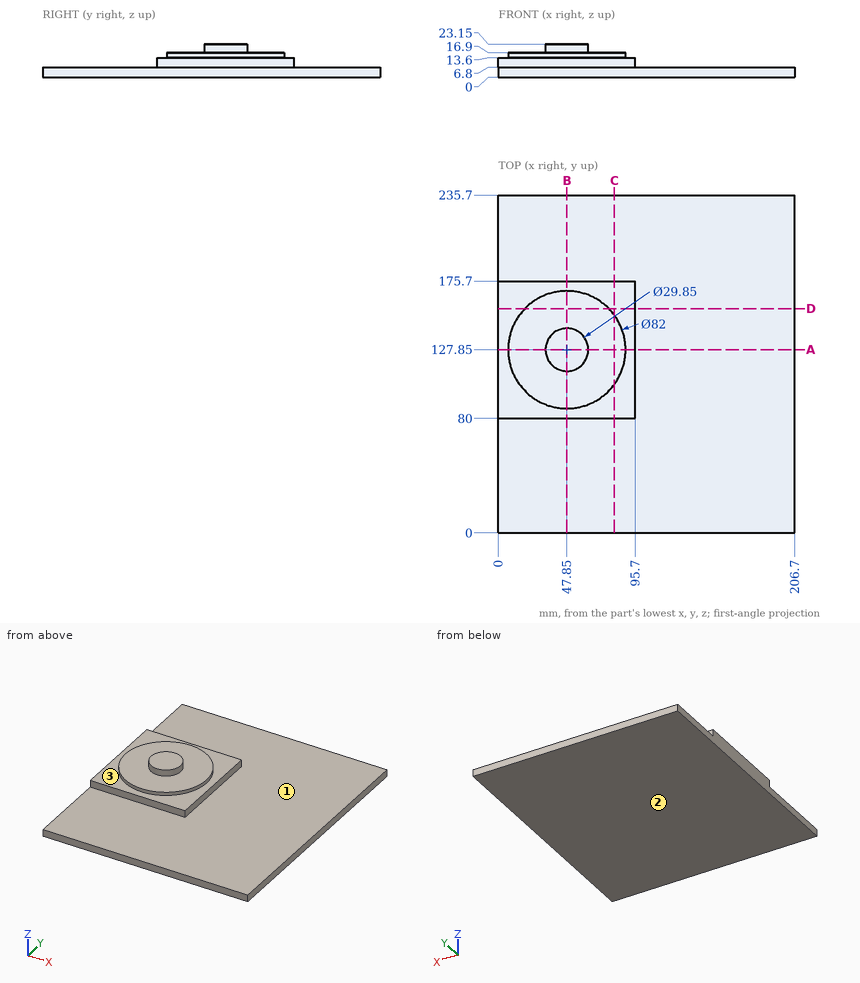
The figure shows three views and two pictorial views of one solid part (mm, origin at its lowest corner). Answer the questions. A direction names the side the tool comes from. Coordinates: 2 decimals unless noted, no trailing zeros. Loops run counter-clockwise (first coordinate to the right, second up) from the corner with the lowest first, then second, coordinate; pieces in that order, holes last.
1) Find section C-C on x = 81. Write down the section's boundary in (y, z), then the cut area to 3 significant figures.
2) Find section D-D on y = 156.5. Write down the section's boundary in (x, z), then the cut area to 3 significant figures.
3) Find section A-A on y = 127.85. Write down the section's boundary in (x, z) (3 decimals), then the cut area to 3 significant figures.
4) Flat-ended cylindrical pins translate along their axes: pin 1 Ø8 at (x, z) = (164, 10.5) entering from -Y; pin 2 Ø12 at (x, z) = (128, 13.5) entering from -Y; pin 3 Ø1.5 at (x, y) = (84, 99.5) entering from +Z; pin 4 Ø2 at (x, z) = (61, 8.5) entering from -Y. Find the tip coordinate at first contact, or state that the pin passes through.
5) A tool of negligible diameter and unlimited length cuts with its end or side. For the marked faces 1, 2 and 3, from which of +Z, -Z, +X, -X, +Y, -Y can it reach the whole face along a straight path? Write none if from no direction.
6) Find section B-B on x = 47.85. Write down the section's boundary in (y, z) (3 decimals).
7) Find the intervals of material crossed by L1, parallel to Z at x = 29.5, y = 98.5; L2, parallel to Z at x = 187, y = 49; L3, parallel to Y at x = 43.5, z = 9.25, in increasing order.
Values:
1. outline: (0, 0) - (235.7, 0) - (235.7, 6.8) - (175.7, 6.8) - (175.7, 13.6) - (151.98, 13.6) - (151.98, 16.9) - (103.72, 16.9) - (103.72, 13.6) - (80, 13.6) - (80, 6.8) - (0, 6.8) - close
1. area: 2,410 mm2
2. outline: (0, 0) - (206.7, 0) - (206.7, 6.8) - (95.7, 6.8) - (95.7, 13.6) - (77.18, 13.6) - (77.18, 16.9) - (18.52, 16.9) - (18.52, 13.6) - (0, 13.6) - close
2. area: 2,250 mm2
3. outline: (0, 0) - (206.7, 0) - (206.7, 6.8) - (95.7, 6.8) - (95.7, 13.6) - (88.85, 13.6) - (88.85, 16.9) - (62.775, 16.9) - (62.775, 23.15) - (32.925, 23.15) - (32.925, 16.9) - (6.85, 16.9) - (6.85, 13.6) - (0, 13.6) - close
3. area: 2,510 mm2
4. pin 1: stops at y = 0
4. pin 2: passes through
4. pin 3: stops at z = 13.6
4. pin 4: stops at y = 80
5. face 1: +Z, +X
5. face 2: -Z, +X, -X, +Y, -Y
5. face 3: +Z
6. outline: (0, 0) - (235.7, 0) - (235.7, 6.8) - (175.7, 6.8) - (175.7, 13.6) - (168.85, 13.6) - (168.85, 16.9) - (142.775, 16.9) - (142.775, 23.15) - (112.925, 23.15) - (112.925, 16.9) - (86.85, 16.9) - (86.85, 13.6) - (80, 13.6) - (80, 6.8) - (0, 6.8) - close
7. L1: z = 0 to 16.9
7. L2: z = 0 to 6.8
7. L3: y = 80 to 175.7
